from build123d import *

# Parameters (mm, degrees)
SKETCH1_R           = 50
SKETCH1_R_2         = 1.8
BOSS_EXTRUDE1_DEPTH = 5
BOSS_EXTRUDE2_START = 5
SKETCH2_R           = 50
SKETCH2_R_2         = 1.8
SKETCH2_R_3         = 6
BOSS_EXTRUDE2_DEPTH = 5


with BuildPart() as part:
    # Sketch1 → Boss-Extrude1 (new body)
    with BuildSketch(Plane(origin=(0, 0, 0), x_dir=(1, 0, 0), z_dir=(0, 1, 0))):
        with Locations(Location((0, 0, 0), (0, 0, 270))):
            Circle(SKETCH1_R)
        with Locations(Location((0, 35, 0), (0, 0, 270))):
            Circle(SKETCH1_R_2, mode=Mode.SUBTRACT)
        with Locations(Location((35, 0, 0), (0, 0, 270))):
            Circle(SKETCH1_R_2, mode=Mode.SUBTRACT)
        with Locations(Location((0, -35, 0), (0, 0, 270))):
            Circle(SKETCH1_R_2, mode=Mode.SUBTRACT)
        with Locations(Location((-35, 0, 0), (0, 0, 270))):
            Circle(SKETCH1_R_2, mode=Mode.SUBTRACT)
        with BuildLine():
            Line((-3.75, 6.5), (-2.47446787, 15.356382884))
            ThreePointArc((-2.47446787, 15.356382884), (0, 17.5), (2.47446787, 15.356382884))
            Line((2.47446787, 15.356382884), (3.75, 6.5))
            Line((3.75, 6.5), (3.754165125, 6.497595264))
            Line((3.754165125, 6.497595264), (12.061783753, 9.821143478))
            ThreePointArc((12.061783753, 9.821143478), (15.155444566, 8.75), (14.536251623, 5.535239406))
            Line((14.536251623, 5.535239406), (7.504165125, 0.002404736))
            Line((7.504165125, 0.002404736), (7.504165125, -0.002404736))
            Line((7.504165125, -0.002404736), (14.536251623, -5.535239406))
            ThreePointArc((14.536251623, -5.535239406), (15.155444566, -8.75), (12.061783753, -9.821143478))
            Line((12.061783753, -9.821143478), (3.754165125, -6.497595264))
            Line((3.754165125, -6.497595264), (3.75, -6.5))
            Line((3.75, -6.5), (2.47446787, -15.356382884))
            ThreePointArc((2.47446787, -15.356382884), (0, -17.5), (-2.47446787, -15.356382884))
            Line((-2.47446787, -15.356382884), (-3.75, -6.5))
            Line((-3.75, -6.5), (-3.754165125, -6.497595264))
            Line((-3.754165125, -6.497595264), (-12.061783753, -9.821143478))
            ThreePointArc((-12.061783753, -9.821143478), (-15.155444566, -8.75), (-14.536251623, -5.535239406))
            Line((-14.536251623, -5.535239406), (-7.504165125, -0.002404736))
            Line((-7.504165125, -0.002404736), (-7.504165125, 0.002404736))
            Line((-7.504165125, 0.002404736), (-14.536251623, 5.535239406))
            ThreePointArc((-14.536251623, 5.535239406), (-15.155444566, 8.75), (-12.061783753, 9.821143478))
            Line((-12.061783753, 9.821143478), (-3.754165125, 6.497595264))
            Line((-3.754165125, 6.497595264), (-3.75, 6.5))
        make_face(mode=Mode.SUBTRACT)
    extrude(amount=BOSS_EXTRUDE1_DEPTH)

    # Sketch2 → Boss-Extrude2 (add)
    with BuildSketch(Plane.XZ.offset(BOSS_EXTRUDE2_START)):
        with Locations(Location((0, 0, 0), (0, 0, 270))):
            Circle(SKETCH2_R)
        with Locations(Location((-35, 0, 0), (0, 0, 270))):
            Circle(SKETCH2_R_2, mode=Mode.SUBTRACT)
        with Locations(Location((0, 35, 0), (0, 0, 270))):
            Circle(SKETCH2_R_2, mode=Mode.SUBTRACT)
        with Locations(Location((35, 0, 0), (0, 0, 270))):
            Circle(SKETCH2_R_2, mode=Mode.SUBTRACT)
        with Locations(Location((0, -35, 0), (0, 0, 270))):
            Circle(SKETCH2_R_2, mode=Mode.SUBTRACT)
        with Locations(Location((0, 0, 0), (0, 0, 270))):
            Circle(SKETCH2_R_3, mode=Mode.SUBTRACT)
    extrude(amount=-BOSS_EXTRUDE2_DEPTH)


solid = part.part
Model file for the job. Use its own axes, mm. A direction names the side the tool comes from. Coordinates: 2 decimals unless noted, no trailing zeros. Loops run counter-clockwise (first coordinate to the right, second up) from the corner with the lowest first, then second, coordinate; pieces in that order, holes last. Notation, with made-up numbers: (-17.75, 67) -> (24.25, 67) arc R16 cw to (24.25, 81) -> close; hole circle Ø3 at (60, 38.5). An arc over 180 degrees is marked (long way). Use one line per item in the form item = value. Start each with the question number.
(1) Cut at A-A on x = 0. Give the cut face in (y, z).
(2) Cut at D-D on x = 35. Give the cut face in (y, z).
(3) Pull direction X, two halves, no side cores. Call faces 3 (the cylindrical face through (15.13, 2.46, -8.79)), 4 (the flat face through (3.12, 2.46, 10.87)), 5 (the flat face through (1, -5, -10)): pulls with the +X half, pulls with the -X half, needs draft (parallel to the pull), parting line crosses it, or undercut.
(4) Tool access for faces 1 (the flat face through (-11.07, 2.46, 2.81)), 2 (the cylindrical face through (1.802, -2.535, -5.723)): list every direction of +Z, -Z, +X, -X, +Y, -Y with a clear straight run to the whole face (end or side of a thin tool).
(5) Probe probe 1 along X at (y, z) = (-2.95, 0); probe 2 along X at (y, z) = (1.35, 0); probe 3 along Z at (x, y) = (0, 2). List the from-to ranges inside material, lowest first. Write a range as from..to.
(6) Cut at B-B on y = 2. Give the number of separate pieces and of enclosed holes in the cut face, and give its area (3 significant figures).
(7) Cut at C-C on z = -35. Give the cut face in (x, y).
(8) Flat gauge pins, fed straight in: pin 1 (6 mm diameter, centred on x = -35, z = 0, fed in from +Y); pin 2 (3 mm diameter, centred on y = 3.5, z = -34, fed in from +X); pin 3 (2 mm diameter, centred on y = 4, z = 39.5, fed in from -X); pin 4 (1 mm diameter, centred on x = -8, y = -1.5, fed in from +Z). Where does each tip first touch, or does it go through?
Values:
q1.outline = (-5, -50) -> (5, -50) -> (5, -36.8) -> (-5, -36.8) -> close; (-5, -33.2) -> (5, -33.2) -> (5, -17.5) -> (0, -17.5) -> (0, -6) -> (-5, -6) -> close; (-5, 6) -> (0, 6) -> (0, 17.5) -> (5, 17.5) -> (5, 33.2) -> (-5, 33.2) -> close; (-5, 36.8) -> (5, 36.8) -> (5, 50) -> (-5, 50) -> close
q2.outline = (-5, -35.71) -> (5, -35.71) -> (5, -1.8) -> (-5, -1.8) -> close; (-5, 1.8) -> (5, 1.8) -> (5, 35.71) -> (-5, 35.71) -> close
q3.face_3 = undercut
q3.face_4 = undercut
q3.face_5 = needs draft
q4.face_1 = +Y
q4.face_2 = +Y, -Y
q5.probe_1 = -50..-36.8, -33.2..-6, 6..33.2, 36.8..50
q5.probe_2 = -50..-36.8, -33.2..-7.5, 7.5..33.2, 36.8..50
q5.probe_3 = -50..-36.8, -33.2..-17.5, 17.5..33.2, 36.8..50
q6.separate_pieces = 1
q6.enclosed_holes = 5
q6.area = 7,290 mm2
q7.outline = (-35.71, -5) -> (-1.8, -5) -> (-1.8, 5) -> (-35.71, 5) -> close; (1.8, -5) -> (35.71, -5) -> (35.71, 5) -> (1.8, 5) -> close
q8.pin_1 = 5
q8.pin_2 = 38
q8.pin_3 = -31.9
q8.pin_4 = 49.43
